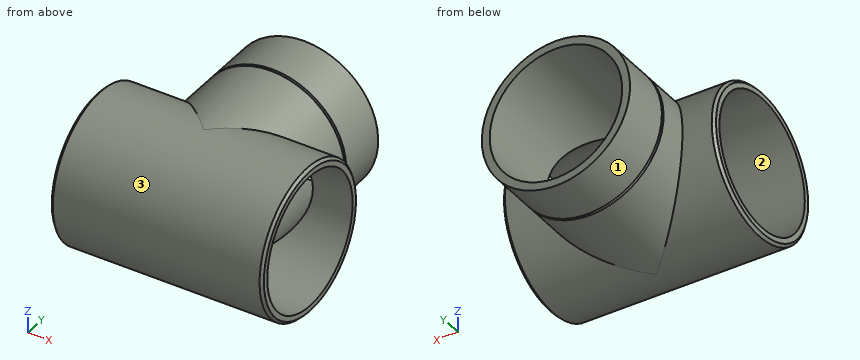
from build123d import *

# Parameters (mm, degrees)
RUNROUTE_R           = 17.9
RUNEXTRUDE_DEPTH     = 25.6
OUTLETROUTE_R        = 17.9
OUTLETEXTRUDE_DEPTH  = 25.6
TEESHELL_START       = -25.6
TEESHELL_OUTLINE_R   = 16
TEESHELL_DEPTH       = 51.2
TEESHELL_START_2     = -1e-07
TEESHELL_2_OUTLINE_R = 16
TEESHELL_2_DEPTH     = 25.6000001
TEECHAMFER_SIZE      = 0.633333333
SKETCH_1_R           = 17.9
SKETCH_1_R_2         = 16
EXTRUDE_1_DEPTH      = 11.933333333


with BuildPart() as part:
    # RunRoute → RunExtrude (new body)
    with BuildSketch(Plane(origin=(0, 0, 0), x_dir=(0, 0, -1), z_dir=(1, 0, 0))):
        Circle(RUNROUTE_R)
    runextrude = extrude(amount=RUNEXTRUDE_DEPTH)

    # RunExtrudeMirror: RunExtrude across plane
    add(runextrude.mirror(Plane(origin=(0, 0, 0), x_dir=(0, 0, 1), z_dir=(1, 0, 0))))

    # OutletRoute → OutletExtrude (add)
    with BuildSketch(Plane(origin=(0, 0, 0), x_dir=(1, 0, 0), z_dir=(0, 1, 0))):
        with Locations(Location((0, 0, 0), (0, 0, 270))):
            Circle(OUTLETROUTE_R)
    extrude(amount=OUTLETEXTRUDE_DEPTH)

    # TeeShell: read off the stored shape, not the designer's step
    # TeeShell outline → TeeShell (cut)
    with BuildSketch(Plane.YZ.offset(TEESHELL_START)):
        Circle(TEESHELL_OUTLINE_R)
    extrude(amount=TEESHELL_DEPTH, mode=Mode.SUBTRACT)

    # TeeShell 2 outline → TeeShell 2 (cut)
    with BuildSketch(Plane(origin=(0, 0, 0), x_dir=(1, 0, 0), z_dir=(0, 1, 0)).offset(TEESHELL_START_2)):
        Circle(TEESHELL_2_OUTLINE_R)
    extrude(amount=TEESHELL_2_DEPTH, mode=Mode.SUBTRACT)

    # TeeChamfer
    # the kernel refuses this chamfer: 0.633333333 mm, written as the material it takes off along each edge
    with BuildSketch(Plane(origin=(25.6, 0, 0), x_dir=(0, 0, -1), z_dir=(0, -1, 0))) as teechamfer_piece_1:
        Polygon((17.9, -TEECHAMFER_SIZE), (17.9 - TEECHAMFER_SIZE, 0), (17.9, 0), align=None)
    revolve(axis=Axis((25.6, 0, 0), (1, 0, 0)), mode=Mode.SUBTRACT)
    with BuildSketch(Plane(origin=(-25.6, 0, 0), x_dir=(0, 0, -1), z_dir=(0, -1, 0))) as teechamfer_piece_2:
        Polygon((17.9, TEECHAMFER_SIZE), (17.9 - TEECHAMFER_SIZE, 0), (17.9, 0), align=None)
    revolve(axis=Axis((-25.6, 0, 0), (1, 0, 0)), mode=Mode.SUBTRACT)
    with BuildSketch(Plane(origin=(0, 25.6, 0), x_dir=(0, 0, 1), z_dir=(-1, 0, 0))) as teechamfer_piece_3:
        Polygon((17.9, -TEECHAMFER_SIZE), (17.9 - TEECHAMFER_SIZE, 0), (17.9, 0), align=None)
    revolve(axis=Axis((0, 25.6, 0), (0, 1, 0)), mode=Mode.SUBTRACT)

    # Эскиз1 → Бобышка-Вытянуть1 (add)
    with BuildSketch(Plane(origin=(0, 25.6, 0), x_dir=(1, 0, 0), z_dir=(0, 1, 0))):
        with Locations(Location((0, 0, 0), (0, 0, 270))):
            Circle(SKETCH_1_R)
        with Locations(Location((0, 0, 0), (0, 0, 270))):
            Circle(SKETCH_1_R_2, mode=Mode.SUBTRACT)
    extrude(amount=EXTRUDE_1_DEPTH)


solid = part.part
Part model, mm, in its own coordinate system. Face numbers are marked on the shaded views. Give positions to 0.01 mm unless a question says otherwise; leave off trailing zeros. Loops run counter-clockwise (first coordinate to the right, second up) from the corner with the lowest first, then second, coordinate; pieces in that order, holes last. Notation, with made-up numbers: M -28.75,75.25 L -5.75,75.25 A25 cw -5.75,99.25 Z; hole C 70.25,20.25 d2. An arc over 180 degrees is marked long. Put each result on its own line as item: value. Start each with the question number.
1) Saw through at B-B (x = 0). List the corners of the cut face in (y, z), then the cut area to 3 significant figures.
2) Flat gauge pins, fed straight in: pin 1 (12 mm diameter, centred on y = 4.5, z = -5.5, fed in from -X); pin 2 (1 mm diameter, centred on x = 4.5, z = 3.5, fed in from -Y); pin 3 (4 mm diameter, centred on x = -18.5, y = 27.5, fed in from +Z); pin 4 (10 mm diameter, centred on x = 2.5, z = 13, fed in from -Y). Where does each tip first touch, or does it go through?
3) Saw through at A-A (z = 0). List the corners of the cut face in (x, y).
4) Saw through at C-C (z = -6). State how many separate pieces and enclosed holes the cut face has, then the cut area to 3 significant figures.
5) Probe probe 1 along X at (y, z) = (20, 0); probe 2 along Z at (x, y) = (-13, 14). List the from-to ranges inside material, lowest first.
6) Pull direction Y, two halves, no side cores. Call the marked faces 1, 2 and 3: +Y half, -Y half, draft (parallel to the pull), parting line (faces both ways), or undercut.
Numbers:
1. outline: M 0,-17.9 L 24.97,-17.9 L 25.6,-17.27 L 25.6,-17.9 L 37.53,-17.9 L 37.53,-16 L 0,-16 A16 cw 0,16 L 37.53,16 L 37.53,17.9 L 25.6,17.9 L 25.6,17.27 L 24.97,17.9 L 0,17.9 A17.9 ccw Z
1. area: 243 mm^2
2. pin 1: through
2. pin 2: y = -17.65
2. pin 3: z = 6.94
2. pin 4: y = -16.01
3. outline: M -25.6,-17.27 L -24.97,-17.9 L 24.97,-17.9 L 25.6,-17.27 L 25.6,-16 L -25.6,-16 Z; M -25.6,16 L -16,16 L -16,37.53 L -17.9,37.53 L -17.9,25.6 L -17.27,25.6 L -17.9,24.97 L -17.9,17.9 L -24.97,17.9 L -25.6,17.27 Z; M 16,16 L 25.6,16 L 25.6,17.27 L 24.97,17.9 L 17.9,17.9 L 17.9,24.97 L 17.27,25.6 L 17.9,25.6 L 17.9,37.53 L 16,37.53 Z
4. separate pieces: 3
4. enclosed holes: 0
4. area: 231 mm^2
5. probe 1: -17.9 to -16, 16 to 17.9
5. probe 2: -12.3 to -9.33, 9.33 to 12.3
6. face 1: draft
6. face 2: undercut
6. face 3: parting line
